Job drawing, mm, ordinate dimensions from the low corner. One solid piece. Give positions to 0.01 mm unless a question says otherwise; leave off trailing zeros. Order: outer loops, then holes, each group sorted by start corner. A loop starts at its lowest first (then second) coordinate and runs counter-clockwise, first axis right, second up.
1. Slice it at A-A on x = 3.35. List the corners of the cut face in (y, z).
2. Drop flat-ended pins along their axis: pin 1 Ø2.5 at (x, y) = (1.5, 3.5) entering from -Z; pin 2 Ø1.5 at (x, y) = (3, 15) entering from +Z; pin 3 Ø2.5 at (x, z) = (3, 131) entering from -Y. Give the stop position or say it passes through.
3. Probe line 1 (Z direction, x = 4.1, y = 80.5); line 2 (Y direction, x = 2.25, z = 79); line 3 (Z direction, x = 0.4, y = 64). List the from-to ranges inside material, lowest first.
4. Slice it at C-C on z = 81.5. List the corners of the cut face in (x, y), and give its area (3 significant figures).
5. Slice it at B-B on y = 72.5. List the corners of the cut face in (x, z).
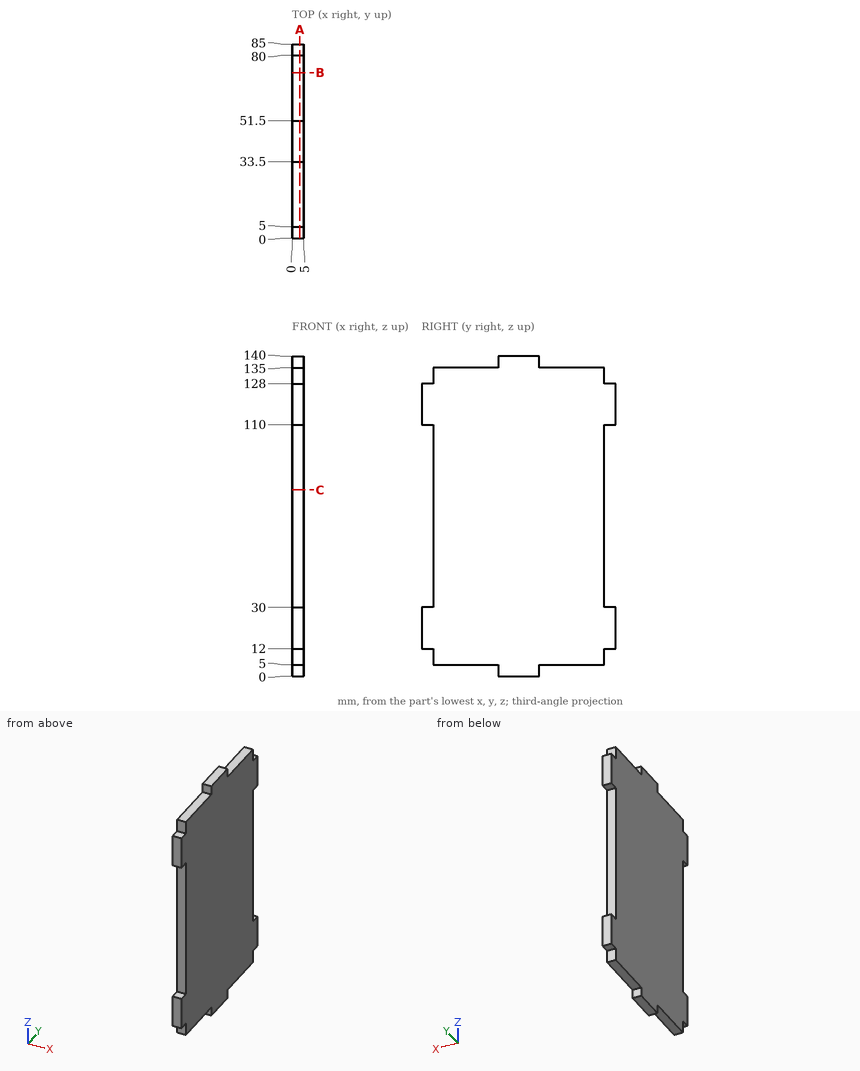
Data:
1. outline: (0, 12) - (5, 12) - (5, 5) - (33.5, 5) - (33.5, 0) - (51.5, 0) - (51.5, 5) - (80, 5) - (80, 12) - (85, 12) - (85, 30) - (80, 30) - (80, 110) - (85, 110) - (85, 128) - (80, 128) - (80, 135) - (51.5, 135) - (51.5, 140) - (33.5, 140) - (33.5, 135) - (5, 135) - (5, 128) - (0, 128) - (0, 110) - (5, 110) - (5, 30) - (0, 30) - close
2. pin 1: stops at z = 12
2. pin 2: stops at z = 135
2. pin 3: stops at y = 5
3. line 1: z = 12 to 30, 110 to 128
3. line 2: y = 5 to 80
3. line 3: z = 5 to 135
4. outline: (0, 5) - (5, 5) - (5, 80) - (0, 80) - close
4. area: 375 mm2
5. outline: (0, 5) - (5, 5) - (5, 135) - (0, 135) - close
